Could you check a few things on this model? Use its own coordinates, in mm. A direction names the side the tool comes from. Round coordinates to 2 decimals unless told otherwise and drop trailing zeros. Write each loop counter-clockwise with the first axis right and the second up, starting at its lowest first coordinate (ties: lowest second). Pieces come first, ordered by that corner, then holes. Notation, with made-up numbers: (-26, 24) -> (27, 24) arc R25 ccw to (27, 47) -> close; hole circle Ø5 at (68.5, -23.75). An arc over 180 degrees is marked (long way). One line per question, with ' | ' between items. Start each with the question number.
1. Imagine slicing it at B-B, the plane x = -14.5. List the corners of the cut face in (y, z) for me, and give its area (3 significant figures).
2. Imagine slicing it at D-D, the plane x = 22.5. List the corners of the cut face in (y, z) for me.
3. If I drill on line 1 along Y through (x, z) = (14.5, -0.7); line 2 along X through (y, z) = (11.75, 2); line 3 along X through (y, z) = (-10, 2.5), over which ranges is the centre line in solid material (lowest first)? Write a range as [from, to].
4. Imagine slicing it at A-A, the plane y = -10. List the corners of the cut face in (x, z) for me, and give its area (3 significant figures).
5. For pin 1 Ø0.5 at (x, z) = (-5.5, -2.5) entering from -Y; pin 2 Ø1.1 at (y, z) = (-7, -2.5) entering from +X; pin 3 Ø3 at (x, y) = (-8, -4.5) entering from -Z, each with a flat end and sliding along its axis, tell me the tip position at first contact or that it passes through.
6. Thinking about a two-plate mould opening in X: for faces 1 (the flat face through (-5.5, -0.5, -2.8)), 2 (the flat face through (-11.5, 0, -3)), 3 (the flat face through (5, 0, -3)), which applies, released by +X, released by -X, zero draft, split by the parting line, or undercut?
7. For faces 4 (the flat face through (20.57, 7, 3)), 5 (the flat face through (-5, 0, -3)), 6 (the flat face through (0, 0.5, -3)), 7 (the flat face through (24, 0.5, 3)), which set-ups out of +Z, -Z, +X, -X, +Y, -Y let a thin tool reach every point of the face, with its end or its side?
from build123d import *

# Parameters (mm, degrees)
F0_W      = 6
F0_H      = 10
F0_R      = 1.55
F0_R_2    = 1.5
F0_W_2    = 10
F0_H_2    = 22
F0_H_3    = 12.5
F0_W_3    = 9
F0_H_4    = 11
F0_H_5    = 2.5
F1_DEPTH  = 1.66
F0_H_6    = 0.5
F2_DEPTH  = 11
F3_DEPTH  = 10.5
F4_R      = 4.49999
F5_R      = 3.25
F6_DEPTH  = 10
F7_DEPTH  = 5.2
F8_R      = 1.5
F9_DEPTH  = 5.1
F10_W     = 1
F10_H     = 1
F11_DEPTH = 2.3


# Not quite as in the source:
# - a fillet or chamfer is up to 0.001 mm smaller than in the source, because OpenCascade refuses the exact size


with BuildPart() as f1:
    # F0 (on Top) → F1 (new body)
    with BuildSketch(Plane.XY):
        Polygon((-27.07, -13.5), (27.07, -13.5), (27.07, 13.5), (10.27, 13.5), (10.27, 11), (10.27, 0), (1.27, 0), (1.27, 11), (1.27, 13.5), (-27.07, 13.5), align=None)
        with Locations((-23.57, -7.75)):
            Rectangle(F0_W, F0_H, mode=Mode.SUBTRACT)
        with Locations((-14.5, -10)):
            Circle(F0_R, mode=Mode.SUBTRACT)
        with Locations((-17.07, 0)):
            Circle(F0_R_2, mode=Mode.SUBTRACT)
        with Locations((-6.07, 0)):
            Rectangle(F0_W_2, F0_H_2, mode=Mode.SUBTRACT)
        with Locations((14.5, -10)):
            Circle(F0_R, mode=Mode.SUBTRACT)
        with Locations((23.57, -6.75)):
            Rectangle(F0_W, F0_H_3, mode=Mode.SUBTRACT)
        with Locations((-23.57, 7.75)):
            Rectangle(F0_W, F0_H, mode=Mode.SUBTRACT)
        with Locations((-14.5, 10)):
            Circle(F0_R, mode=Mode.SUBTRACT)
        with Locations((23.57, 6.75)):
            Rectangle(F0_W, F0_H_3, mode=Mode.SUBTRACT)
        with Locations((14.5, 10)):
            Circle(F0_R, mode=Mode.SUBTRACT)
        with Locations((-6.07, 0)):
            Rectangle(F0_W_2, F0_H_2)
        with Locations((5.77, 5.5)):
            Rectangle(F0_W_3, F0_H_4)
        with Locations((23.57, 6.75)):
            Rectangle(F0_W, F0_H_3)
        with Locations((23.57, -6.75)):
            Rectangle(F0_W, F0_H_3)
        with Locations((-23.57, 7.75)):
            Rectangle(F0_W, F0_H)
        with Locations((-23.57, -7.75)):
            Rectangle(F0_W, F0_H)
        with Locations((5.77, 12.25)):
            Rectangle(F0_W_3, F0_H_5)
        with Locations((-17.07, 0)):
            Circle(F0_R_2)
    extrude(amount=-F1_DEPTH)

    # F0 (on Top) → F2 (join)
    with BuildSketch(Plane.XY):
        with Locations((5.77, 12.25)):
            Rectangle(F0_W_3, F0_H_5)
        with Locations((5.77, 13.75)):
            Rectangle(F0_W_3, F0_H_6)
    extrude(amount=F2_DEPTH)

    # F0 (on Top) → F3 (join)
    with BuildSketch(Plane.XY):
        with Locations((5.77, 5.5)):
            Rectangle(F0_W_3, F0_H_4)
    extrude(amount=F3_DEPTH)

    # F4 (radius 4.5 in the source; OpenCascade refuses exactly that, so slightly less here)
    f4_edges = [f1.edges().sort_by_distance(p)[0] for p in [
        (1.27, 5.5, 10.5),
        (10.27, 5.5, 10.5),
    ]]
    fillet(f4_edges, radius=F4_R)

    # F5 (on face) → F6 (cut)
    with BuildSketch(Plane(origin=(0, 14, 0), x_dir=(-1, 0, 0), z_dir=(0, 1, 0))):
        with Locations((-5.77, 6.3)):
            Circle(F5_R)
    extrude(amount=-F6_DEPTH, mode=Mode.SUBTRACT)

    # F0 (on Top) → F7 (join)
    with BuildSketch(Plane.XY):
        with Locations((-17.07, 0)):
            Circle(F0_R_2)
    extrude(amount=F7_DEPTH)

    # F8
    f8_edges = [f1.edges().sort_by_distance(p)[0] for p in [
        (-18.57, 0, 5.2),
    ]]
    fillet(f8_edges, radius=F8_R)

    # F0 (on Top) → F9 (join)
    with BuildSketch(Plane.XY):
        with Locations((23.57, 6.75)):
            Rectangle(F0_W, F0_H_3)
        with Locations((23.57, -6.75)):
            Rectangle(F0_W, F0_H_3)
        with Locations((-23.57, -7.75)):
            Rectangle(F0_W, F0_H)
        with Locations((-23.57, 7.75)):
            Rectangle(F0_W, F0_H)
    extrude(amount=F9_DEPTH)

    # F10 (on face) → F11 (join)
    with BuildSketch(Plane(origin=(0, 0, -1.66), x_dir=(1, 0, 0), z_dir=(0, 0, -1))):
        Rectangle(F10_W, F10_H)
        with Locations((0, 7)):
            Rectangle(F10_W, F10_H)
        with Locations((5.5, 7)):
            Rectangle(F10_W, F10_H)
        with Locations((11, 7)):
            Rectangle(F10_W, F10_H)
        with Locations((11, 0)):
            Rectangle(F10_W, F10_H)
        with Locations((5.5, 0)):
            Rectangle(F10_W, F10_H)
        with Locations((11, -7)):
            Rectangle(F10_W, F10_H)
        with Locations((5.5, -7)):
            Rectangle(F10_W, F10_H)
        with Locations((0, -7)):
            Rectangle(F10_W, F10_H)
        with Locations((-5.5, -7)):
            Rectangle(F10_W, F10_H)
        with Locations((-5.5, 0)):
            Rectangle(F10_W, F10_H)
        with Locations((-5.5, 7)):
            Rectangle(F10_W, F10_H)
        with Locations((-11, 7)):
            Rectangle(F10_W, F10_H)
        with Locations((-11, 0)):
            Rectangle(F10_W, F10_H)
        with Locations((-11, -7)):
            Rectangle(F10_W, F10_H)
    extrude(amount=F11_DEPTH)


solid = f1.part
Geometry results:
1) outline: (-13.5, -1.66) -> (-11.55, -1.66) -> (-11.55, 0) -> (-13.5, 0) -> close; (-8.45, -1.66) -> (8.45, -1.66) -> (8.45, 0) -> (-8.45, 0) -> close; (11.55, -1.66) -> (13.5, -1.66) -> (13.5, 0) -> (11.55, 0) -> close | area: 34.5 mm2
2) outline: (-13.5, -1.66) -> (13.5, -1.66) -> (13.5, 0) -> (13, 0) -> (13, 5.1) -> (0.5, 5.1) -> (0.5, 0) -> (-0.5, 0) -> (-0.5, 5.1) -> (-13, 5.1) -> (-13, 0) -> (-13.5, 0) -> close
3) line 1: y = [-13.5, -11.55], [-8.45, 8.45], [11.55, 13.5] | line 2: x = [-26.57, -20.57], [1.27, 10.27], [20.57, 26.57] | line 3: x = [-26.57, -20.57], [20.57, 26.57]
4) outline: (-27.07, -1.66) -> (-16.05, -1.66) -> (-16.05, 0) -> (-20.57, 0) -> (-20.57, 5.1) -> (-26.57, 5.1) -> (-26.57, 0) -> (-27.07, 0) -> close; (-12.95, -1.66) -> (12.95, -1.66) -> (12.95, 0) -> (-12.95, 0) -> close; (16.05, -1.66) -> (27.07, -1.66) -> (27.07, 0) -> (26.57, 0) -> (26.57, 5.1) -> (20.57, 5.1) -> (20.57, 0) -> (16.05, 0) -> close | area: 141 mm2
5) pin 1: stops at y = -7.5 | pin 2: stops at x = 11.5 | pin 3: stops at z = -1.66
6) face 1: zero draft | face 2: released by -X | face 3: undercut
7) face 4: +Z, +Y, -Y | face 5: -Z, +Y, -Y | face 6: -Z, +X, -X | face 7: +Z, +X
